```python
from build123d import *

# Parameters (mm, degrees)
BOSS_EXTRUDE2_DEPTH  = 12
BOSS_EXTRUDE3_START  = -12
BOSS_EXTRUDE3_DEPTH  = 12
CUT_EXTRUDE6_START   = -4
CUT_EXTRUDE6_DEPTH   = 4
CUT_EXTRUDE7_REACH   = 18.348
SKETCH4_R            = 0.975
MIRROR2_START        = -4
MIRROR2_COPY_1_DEPTH = 4


# Read off the part's stored shape, not the designer's step: Boss-Extrude3
with BuildPart() as part:
    # Sketch1 → Boss-Extrude2 (new body)
    with BuildSketch(Plane.XY):
        with BuildLine():
            Line((0, 6), (0, 7.5))
            ThreePointArc((0, 7.5), (-3.75510396, 6.492241081), (-6.501077384, 3.739785134))
            Line((-6.501077384, 3.739785134), (-6.501077384, -3.739785134))
            ThreePointArc((-6.501077384, -3.739785134), (-3.75510396, -6.492241081), (0, -7.5))
            Line((0, -7.5), (0, -6))
            ThreePointArc((0, -6), (-2.838133189, -5.286303056), (-5.001077384, -3.315))
            ThreePointArc((-5.001077384, -3.315), (-6, 0), (-5.001077384, 3.315))
            ThreePointArc((-5.001077384, 3.315), (-2.838133189, 5.286303056), (0, 6))
        make_face()
        with BuildLine():
            Line((-5.001077384, -3.315), (-5.001077384, 3.315))
            ThreePointArc((-5.001077384, 3.315), (-6, 0), (-5.001077384, -3.315))
        make_face()
    extrude(amount=BOSS_EXTRUDE2_DEPTH)

    # Boss-Extrude3 outline → Boss-Extrude3 (add)
    with BuildSketch(Plane.XY.offset(12).offset(BOSS_EXTRUDE3_START)):
        with BuildLine():
            ThreePointArc((-3.5, 6.633249581), (-1.802862744, 7.280088319), (0, 7.5))
            Line((0, 7.5), (0, 9))
            Line((0, 9), (-3.5, 9))
            Line((-3.5, 9), (-3.5, 6.633249581))
        make_face()
    boss_extrude3 = extrude(amount=BOSS_EXTRUDE3_DEPTH)

    # Sketch3 → Cut-Extrude6 (cut)
    with BuildSketch(Plane.XY.offset(12).offset(CUT_EXTRUDE6_START)):
        with BuildLine():
            Line((-4.617876388, 10.846765639), (-4.617876388, 5.909756142))
            ThreePointArc((-4.617876388, 5.909756142), (-1.858071818, 7.266193578), (1.214101671, 7.401078106))
            Line((1.214101671, 7.401078106), (1.214101671, 10.846765639))
            Line((1.214101671, 10.846765639), (-4.617876388, 10.846765639))
        make_face()
    cut_extrude6 = extrude(amount=CUT_EXTRUDE6_DEPTH, mode=Mode.SUBTRACT)

    # Mirror1: Cut-Extrude6 across plane
    add(cut_extrude6.mirror(Plane.XY.offset(6)), mode=Mode.SUBTRACT)

    # Sketch4 → Cut-Extrude7 (cut, up to next)
    with BuildSketch(Plane(origin=(0, 0, 0), x_dir=(0, 0, -1), z_dir=(1, 0, 0)), mode=Mode.PRIVATE) as cut_extrude7_sk1:
        with Locations((-6, 7.75)):
            Circle(SKETCH4_R)
    cut_extrude7_tool1 = extrude(cut_extrude7_sk1.sketch, amount=-CUT_EXTRUDE7_REACH, mode=Mode.PRIVATE) & part.part
    cut_extrude7 = cut_extrude7_tool1.solids().sort_by_distance((0, 7.75, 6))[0]
    add(cut_extrude7, mode=Mode.SUBTRACT)

    # Mirror2: Boss-Extrude3, Cut-Extrude6, Cut-Extrude7 across plane
    add(boss_extrude3.mirror(Plane.ZX))
    add(cut_extrude6.mirror(Plane.ZX), mode=Mode.SUBTRACT)
    add(cut_extrude7.mirror(Plane.ZX), mode=Mode.SUBTRACT)

    # Mirror2 copy 1 sketch → Mirror2 copy 1 (cut)
    with BuildSketch(Plane(origin=(0, 0, 0), x_dir=(1, 0, 0), z_dir=(0, 0, -1)).offset(MIRROR2_START)):
        with BuildLine():
            Line((-4.617876388, 10.846765639), (-4.617876388, 5.909756142))
            ThreePointArc((-4.617876388, 5.909756142), (-1.858071818, 7.266193578), (1.214101671, 7.401078106))
            Line((1.214101671, 7.401078106), (1.214101671, 10.846765639))
            Line((1.214101671, 10.846765639), (-4.617876388, 10.846765639))
        make_face()
    extrude(amount=MIRROR2_COPY_1_DEPTH, mode=Mode.SUBTRACT)


solid = part.part
```
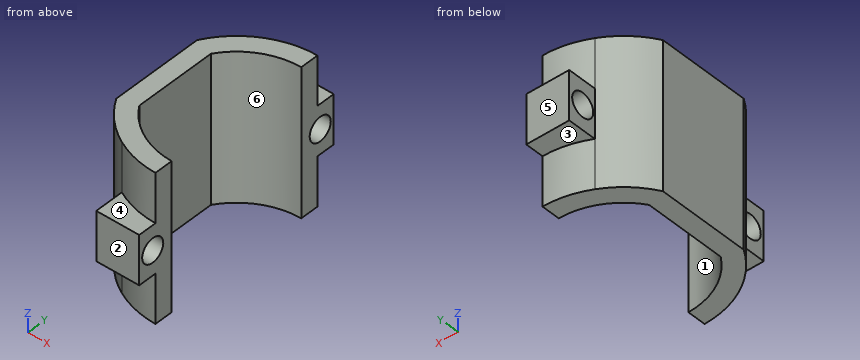
Check sheet for the modelled part. Datum: model origin and axes. Units: mm. Face numbers are marked on the shaded views. A direction names the side the tool comes from. Round coordinates to 2 decimals unless told otherwise and drop trailing zeros. Loops run counter-clockwise (first coordinate to the right, second up) from the corner with the lowest first, then second, coordinate; pieces in that order, holes last. Notation, with made-up numbers: (-15.75, -14) -> (2.25, -14) arc R20 ccw to (2.25, 10) -> close; hole circle Ø7 at (-8.5, 65.5). An arc over 180 degrees is marked (long way). Answer in a Markdown table with one row per item.
Q1. Set-up check for the marked faces 1, 2 and 3: record each of +Z, -Z, +X, -X, +Y, -Y from which the full face is reachable in a straight line by a thin tool's end or side.
Data:
| item | result |
|---|---|
| face 1 | +Z, -Z, +X |
| face 2 | +Z, -Z, +X, -X, -Y |
| face 3 | -Z, -X, +Y |
Q2. Sectioned sample at D-D on z = 4.75. Enter the section's corners in (x, y) (3 decimals), then the cut area to 3 significant figures.
Data:
| item | result |
|---|---|
| outline | (-6.501, -3.74) arc R7.5 ccw to (-3.5, -6.633) -> (-3.5, -9) -> (0, -9) -> (0, -6) arc R6 cw to (-5.001, -3.315) -> (-5.001, 3.315) arc R6 cw to (0, 6) -> (0, 9) -> (-3.5, 9) -> (-3.5, 6.633) arc R7.5 ccw to (-6.501, 3.74) -> close |
| area | 43.7 mm^2 |
Q3. Sectioned sample at A-A on y = 7.75. Enter the section's corners in (x, z) (3 decimals).
Data:
| item | result |
|---|---|
| outline | (-3.5, 4) -> (0, 4) -> (0, 5.025) -> (-3.5, 5.025) -> close; (-3.5, 6.975) -> (0, 6.975) -> (0, 8) -> (-3.5, 8) -> close |
Q4. Sectioned sample at C-C on x = -4.25. Enter the section's corners in (y, z), then the cut area to 3 significant figures.
Data:
| item | result |
|---|---|
| outline | (-6.18, 0) -> (-4.24, 0) -> (-4.24, 12) -> (-6.18, 12) -> close; (4.24, 0) -> (6.18, 0) -> (6.18, 12) -> (4.24, 12) -> close |
| area | 46.7 mm^2 |
Q5. Thickness scan on L1, parallel to Y at x = -1.75, z = 6 (3 decimals); L2, parallel to Z at x = -1.4, y = -7.75 (3 decimals); L3, parallel to Y at x = -1, z = 6 (3 decimals). Record the ranges inside material, lowest first.
Data:
| item | result |
|---|---|
| L1 | y = -9 to -8.725, -6.775 to -5.739, 5.739 to 6.775, 8.725 to 9 |
| L2 | z = 4 to 5.025, 6.975 to 8 |
| L3 | y = -9 to -8.725, -6.775 to -5.916, 5.916 to 6.775, 8.725 to 9 |
Q6. Go/stop test with flat-tipped pins: P1, Ø2.5, axis at y = 7.75, z = 6, coming from the -X side; P2, Ø5, axis at y = -1, z = 1.5, coming from the +X side; P3, Ø3.5, axis at y = 1.5, z = 7.5, coming from the +X side. Record where each tip stops, or that it passes through.
Data:
| item | result |
|---|---|
| P1 | stops at x = -3.74 |
| P2 | stops at x = -4.87 |
| P3 | stops at x = -5 |
Q7. Release check for a two-part mould opening along Y. For the marked faces 4, 5 and 6 record: released by +Y, released by -Y, zero draft, split by the parting line, or undercut.
Data:
| item | result |
|---|---|
| face 4 | zero draft |
| face 5 | released by +Y |
| face 6 | undercut |
Q8. Sectioned sample at B-B on z = 6. Enter the section's corners in (x, y) (3 decimals), then the cut area to 3 significant figures.
Data:
| item | result |
|---|---|
| outline | (-6.501, -3.74) arc R7.5 ccw to (-3.5, -6.633) -> (-3.5, -6.775) -> (0, -6.775) -> (0, -6) arc R6 cw to (-5.001, -3.315) -> (-5.001, 3.315) arc R6 cw to (0, 6) -> (0, 6.775) -> (-3.5, 6.775) -> (-3.5, 6.633) arc R7.5 ccw to (-6.501, 3.74) -> close; (-3.5, -9) -> (0, -9) -> (0, -8.725) -> (-3.5, -8.725) -> close; (-3.5, 8.725) -> (0, 8.725) -> (0, 9) -> (-3.5, 9) -> close |
| area | 30.1 mm^2 |
